Autodesk Inventor part; units mm, degrees
ref_plane "Work Plane1" through (0, 0, -83.82) normal (0, 0, 1) x (1, 0, 0)
ref_plane "Work Plane2" through (0, 4.826, 0) normal (0, 1, 0) x (-1, 0, 0)
ref_plane "Work Plane3" through (4.826, 0, 0) normal (1, 0, 0) x (0, 1, 0)
sketch "Sketch1" plane through (0, 0, 0) normal (0, 0, 1) x (1, 0, 0)
  point P0 (0, 0)
sketch "Sketch2" plane through (0, 0, 0) normal (0, 0, 1) x (1, 0, 0)
  circle A0 centre (0, 0) radius 3.683
  dimension "d0" = 7.366
ref_plane "Work Plane1" through (0, 0, -83.82) normal (0, 0, 1) x (1, 0, 0)
sketch "Sketch3" plane through (0, 0, -83.82) normal (0, 0, 1) x (1, 0, 0)
  circle A0 centre (0, 0) radius 4.826
  dimension "d2" = 9.652
loft "Loft1" add profiles "Sketch2", "Sketch3"
fillet "Fillet1" radius 1.5875 1 edges at (-3.683, 0, 0)
ref_plane "Work Plane2" through (0, 4.826, 0) normal (0, 1, 0) x (-1, 0, 0)
sketch "Sketch4" plane through (0, 4.826, 0) normal (0, 1, 0) x (-1, 0, 0)
  circle A0 centre (0, -78.74) radius 0.8255
  line L0 (4.826, -83.82) -> (-4.826, -83.82)
  point P0 (0, 0)
  dimension "d9" = 1.651
  dimension "d10" = 5.08
extrude "Extrusion1" cut sketch "Sketch4" against normal up to next
ref_plane "Work Plane3" through (4.826, 0, 0) normal (1, 0, 0) x (0, 1, 0)
sketch "Sketch8" plane through (4.826, 0, 0) normal (1, 0, 0) x (0, 1, 0)
  line L0 (4.826, -83.82) -> (-4.826, -83.82)
  line L1 (-2.794, -74.041) -> (2.794, -74.041)
  line L2 (2.794, -74.041) -> (2.794, -83.82)
  line L3 (2.794, -83.82) -> (-2.794, -83.82)
  line L4 (-2.794, -83.82) -> (-2.794, -74.041)
  point P0 (0, 0)
  dimension "d14" = 2.794
  dimension "d15" = 5.588
  dimension "d16" = 9.779
extrude "Extrusion2" cut sketch "Sketch8" against normal blind 6.096
properties part number "AntennaMast"
Can you work these out from the model? Positions are in its coordinate system, mm. A direction names the side the tool comes from. Round coordinates to 2 decimals unless told otherwise and drop trailing zeros. Loops run counter-clockwise (first coordinate to the right, second up) from the corner with the lowest first, then second, coordinate; pieces in that order, holes last. Notation, with made-up numbers: (21.5, -30.5) -> (78.5, -30.5) arc R18 ccw to (78.5, -10.5) -> close; hole circle Ø7 at (30, 55). An arc over 180 degrees is marked (long way). Answer in a Markdown table with one row per item.
Item 1: We'd pull the mould along X, two halves only. Please class faces 1 (the flat face through (-1.27, 0, -79)), 2 (the flat face through (-1.5, 0.1, -83.82)), 3 (the cylindrical face through (0.11, -3.77, -77.92)), 4 (the cylindrical face through (0.11, 3.79, -77.92)): released by +X, released by -X, zero draft, split by the parting line, or undercut.
Answer block:
| item | result |
|---|---|
| face 1 | released by +X |
| face 2 | zero draft |
| face 3 | undercut |
| face 4 | undercut |
Item 2: Suppose I cut it at D-D, the plane z = -44.5. List the corners of the cut face in (x, y) for me, plus the area to 3 significant figures.
Answer block:
| item | result |
|---|---|
| outline | circle Ø8.58 at (0, 0) |
| area | 57.8 mm² |
Item 3: Suppose I cut it at C-C, the plane z = -58. List the corners of the cut face in (x, y) for me.
Answer block:
| item | result |
|---|---|
| outline | circle Ø8.95 at (0, 0) |
Item 4: Will these pins go through, and if not, where does the flat tip stop? P1, Ø2, axis at x = 0, z = -78.74, coming from the +Y side; P2, Ø4, axis at x = 2.5, z = -49.5, coming from the +Y side; P3, Ø4, axis at x = 0.5, z = -79.5, coming from the -Y side.
Answer block:
| item | result |
|---|---|
| P1 | y = 4.77 |
| P2 | y = 4.33 |
| P3 | y = -4.79 |
Item 5: On a 3-axis mill with a long thin cutter (end or side, diameter ignored), from which of +Z, -Z, +X, -X, +Y, -Y can I reach the whole of each face in a straight line? I mean faces 5 (the flat face through (0, 0, 0)), 6 (the conical face through (-4.27, -0.19, -43.27)), 7 (the flat face through (2, 0, -74.041)). Say none if no direction works.
Answer block:
| item | result |
|---|---|
| face 5 | +Z, +X, -X, +Y, -Y |
| face 6 | +Z |
| face 7 | -Z, +X |
Item 6: If I drill on probe 1 along Z at (x, y) = (-1, -1.75); probe 2 along X at (y, z) = (-3.85, -78.74); probe 3 along Z at (x, y) = (0, 3.25), over which ranges is the centre line in solid material (lowest first)?
Answer block:
| item | result |
|---|---|
| probe 1 | -74.04 to 0 |
| probe 2 | -2.79 to -0.83, 0.83 to 2.79 |
| probe 3 | -83.82 to -79.57, -77.91 to -0.48 |
Item 7: Suppose I cut it at B-B, the plane x = 0. Give the number of separate pieces and of enclosed holes in the cut face, plus the area to 3 significant figures.
Answer block:
| item | result |
|---|---|
| separate pieces | 3 |
| enclosed holes | 0 |
| area | 651 mm² |
Item 8: Suppose I cut it at A-A, the plane z = -78.74. List the corners of the cut face in (x, y) for me.
Answer block:
| item | result |
|---|---|
| outline | (-1.27, -2.79) -> (-1.27, 2.79) -> (-0.83, 2.79) -> (-0.83, 4.68) arc R4.76 ccw to (-0.83, -4.68) -> (-0.83, -2.79) -> close; (0.83, -4.68) arc R4.76 ccw to (3.85, -2.79) -> (0.83, -2.79) -> close; (0.83, 2.79) -> (3.85, 2.79) arc R4.76 ccw to (0.83, 4.68) -> close |
